from build123d import *

# Parameters (mm, degrees)
SKETCH1_W                    = 80
SKETCH1_H                    = 80
PCB_DEPTH                    = 2
SKETCH7_W                    = 33
SKETCH7_H                    = 35
LIPO_ADAFRUIT_CHARGERS_DEPTH = 5
LPATTERN2_COUNT              = 2
LPATTERN2_PITCH              = 47
LPATTERN2_COUNT_DIR2         = 2
LPATTERN2_PITCH_DIR2         = 45
SKETCH4_R                    = 1.8
ATTACHMENT_HOLES_DEPTH       = 6
ATTACHMENT_HOLES_DEPTH_BACK  = 3
SKETCH8_R                    = 1.5875
CUT_EXTRUDE1_DEPTH           = 8
LPATTERN3_COUNT              = 2
LPATTERN3_PITCH              = 70
LPATTERN3_COUNT_DIR2         = 2
LPATTERN3_PITCH_DIR2         = 20
SKETCH9_R                    = 1.5875
CUT_EXTRUDE2_DEPTH           = 8


with BuildPart() as part:
    # Sketch1 → PCB (new body)
    with BuildSketch(Plane(origin=(0, 0, 0), x_dir=(1, 0, 0), z_dir=(0, 1, 0))):
        with Locations((40, 40)):
            Rectangle(SKETCH1_W, SKETCH1_H)
    extrude(amount=PCB_DEPTH)

    # Sketch7 → LiPo Adafruit Chargers (add)
    with BuildSketch(Plane(origin=(0, 2, 0), x_dir=(1, 0, 0), z_dir=(0, 1, 0))):
        with Locations((63.5, 17.5)):
            Rectangle(SKETCH7_W, SKETCH7_H)
    lipo_adafruit_chargers = extrude(amount=LIPO_ADAFRUIT_CHARGERS_DEPTH)

    # LPattern2: LiPo Adafruit Chargers 2 × 2
    with Locations(*[(-i * LPATTERN2_PITCH, 0, -j * LPATTERN2_PITCH_DIR2) for i in range(LPATTERN2_COUNT) for j in range(LPATTERN2_COUNT_DIR2) if (i, j) != (0, 0)]):
        add(lipo_adafruit_chargers)

    # Sketch4 → Attachment holes (cut, two sides)
    with BuildSketch(Plane(origin=(0, 2, 0), x_dir=(1, 0, 0), z_dir=(0, 1, 0))) as attachment_holes_sk:
        with Locations((5, 75)):
            Circle(SKETCH4_R)
        with Locations((75, 75)):
            Circle(SKETCH4_R)
        with Locations((75, 5)):
            Circle(SKETCH4_R)
        with Locations((5, 5)):
            Circle(SKETCH4_R)
    extrude(amount=ATTACHMENT_HOLES_DEPTH, mode=Mode.SUBTRACT)
    extrude(attachment_holes_sk.sketch, amount=-ATTACHMENT_HOLES_DEPTH_BACK, mode=Mode.SUBTRACT)

    # Sketch8 → Cut-Extrude1 (cut, through all)
    with BuildSketch(Plane(origin=(0, 7, 0), x_dir=(1, 0, 0), z_dir=(0, 1, 0))):
        with Locations((5, 30)):
            Circle(SKETCH8_R)
    cut_extrude1 = extrude(amount=-CUT_EXTRUDE1_DEPTH, mode=Mode.SUBTRACT)

    # LPattern3: Cut-Extrude1 2 × 2
    with Locations(*[(i * LPATTERN3_PITCH, 0, -j * LPATTERN3_PITCH_DIR2) for i in range(LPATTERN3_COUNT) for j in range(LPATTERN3_COUNT_DIR2) if (i, j) != (0, 0)]):
        add(cut_extrude1, mode=Mode.SUBTRACT)

    # Sketch9 → Cut-Extrude2 (cut, through all)
    with BuildSketch(Plane(origin=(0, 7, 0), x_dir=(1, 0, 0), z_dir=(0, 1, 0))):
        with Locations((28, 5)):
            Circle(SKETCH9_R)
    extrude(amount=-CUT_EXTRUDE2_DEPTH, mode=Mode.SUBTRACT)


solid = part.part
Model file for the job. Use its own axes, mm. A direction names the side the tool comes from. Coordinates: 2 decimals unless noted, no trailing zeros. Order: outer loops, then holes, each group sorted by start corner. A loop starts at its lowest first (then second) coordinate and runs counter-clockwise, first axis right, second up. Notation, with made-up numbers: (44.25, -10.5) -> (76.25, -10.5) arc R6 ccw to (76.25, -2.5) -> close; hole circle Ø11 at (28, -37). An arc over 180 degrees is marked (long way). Return JSON: item names as keys, results as strings. Group by question number.
Item 1: Saw through at B-B on x = 5. Write the cut outline in (y, z).
Item 2: Tool access for faces 4 (the flat face through (63, 7, -18)), 5 (the flat face through (63, 4, -45)), 6 (the flat face through (33, 4, -17)): list every direction of +Z, -Z, +X, -X, +Y, -Y with a clear straight run to the whole face (end or side of a thin tool).
Item 3: Saw through at D-D on z = -50. Write the cut outline in (x, y), then the cut area to 3 significant figures.
Item 4: Flat gauge pin, fed straight in: P1, Ø2, axis at x = 35.5, y = 5, coming from the +Z side. Where does the tip first touch, or does it go through?
Item 5: Saw through at A-A on y = 4.75. State how many separate pieces and enclosed holes the cut face has, then the cut area to 3 significant figures.
Item 6: Wall check: line 1 along X through (y, z) = (5.7, -75); line 2 along X through (y, z) = (3.5, -30); line 3 along Z through (x, y) = (75, 1). Give the ranges that are in metal, low to high. Write a range as [from, to].
Item 7: Pull direction X, two halves, no side cores. Call faces 1 (the flat face through (80, 1, -39)), 2 (the flat face through (47, 4, -62)), 3 (the flat face through (16, 4, -35)): pulls with the +X half, pulls with the -X half, needs draft (parallel to the pull), parting line crosses it, or undercut.
Item 8: Saw through at C-C on z = -5. Write the cut outline in (x, y), then the cut area to 3 significant figures.
Values found:
{
 "1": {"outline": "(0, -80) -> (7, -80) -> (7, -76.8) -> (0, -76.8) -> close; (0, -73.2) -> (7, -73.2) -> (7, -51.59) -> (0, -51.59) -> close; (0, -48.41) -> (7, -48.41) -> (7, -45) -> (2, -45) -> (2, -35) -> (7, -35) -> (7, -31.59) -> (0, -31.59) -> close; (0, -28.41) -> (7, -28.41) -> (7, -6.8) -> (0, -6.8) -> close; (0, -3.2) -> (7, -3.2) -> (7, 0) -> (0, 0) -> close"},
 "2": {"face 4": "+Z, -Z, +X, -X, +Y", "face 5": "+X, -X, +Y", "face 6": "+Z, -Z, +Y"},
 "3": {"outline": "(0, 0) -> (3.41, 0) -> (3.41, 7) -> (0, 7) -> close; (6.59, 0) -> (73.41, 0) -> (73.41, 7) -> (47, 7) -> (47, 2) -> (33, 2) -> (33, 7) -> (6.59, 7) -> close; (76.59, 0) -> (80, 0) -> (80, 7) -> (76.59, 7) -> close", "area": "446 mm2"},
 "4": {"P1": "passes through"},
 "5": {"separate pieces": "4", "enclosed holes": "9", "area": "4,540 mm2"},
 "6": {"line 1": "x = [0, 3.2], [6.8, 33], [47, 73.2], [76.8, 80]", "line 2": "x = [0, 3.41], [6.59, 33], [47, 73.41], [76.59, 80]", "line 3": "z = [-80, -76.8], [-73.2, -51.59], [-48.41, -31.59], [-28.41, -6.8], [-3.2, 0]"},
 "7": {"face 1": "pulls with the +X half", "face 2": "undercut", "face 3": "needs draft"},
 "8": {"outline": "(0, 0) -> (3.2, 0) -> (3.2, 7) -> (0, 7) -> close; (6.8, 0) -> (26.41, 0) -> (26.41, 7) -> (6.8, 7) -> close; (29.59, 0) -> (73.2, 0) -> (73.2, 7) -> (47, 7) -> (47, 2) -> (33, 2) -> (33, 7) -> (29.59, 7) -> close; (76.8, 0) -> (80, 0) -> (80, 7) -> (76.8, 7) -> close", "area": "417 mm2"}
}
